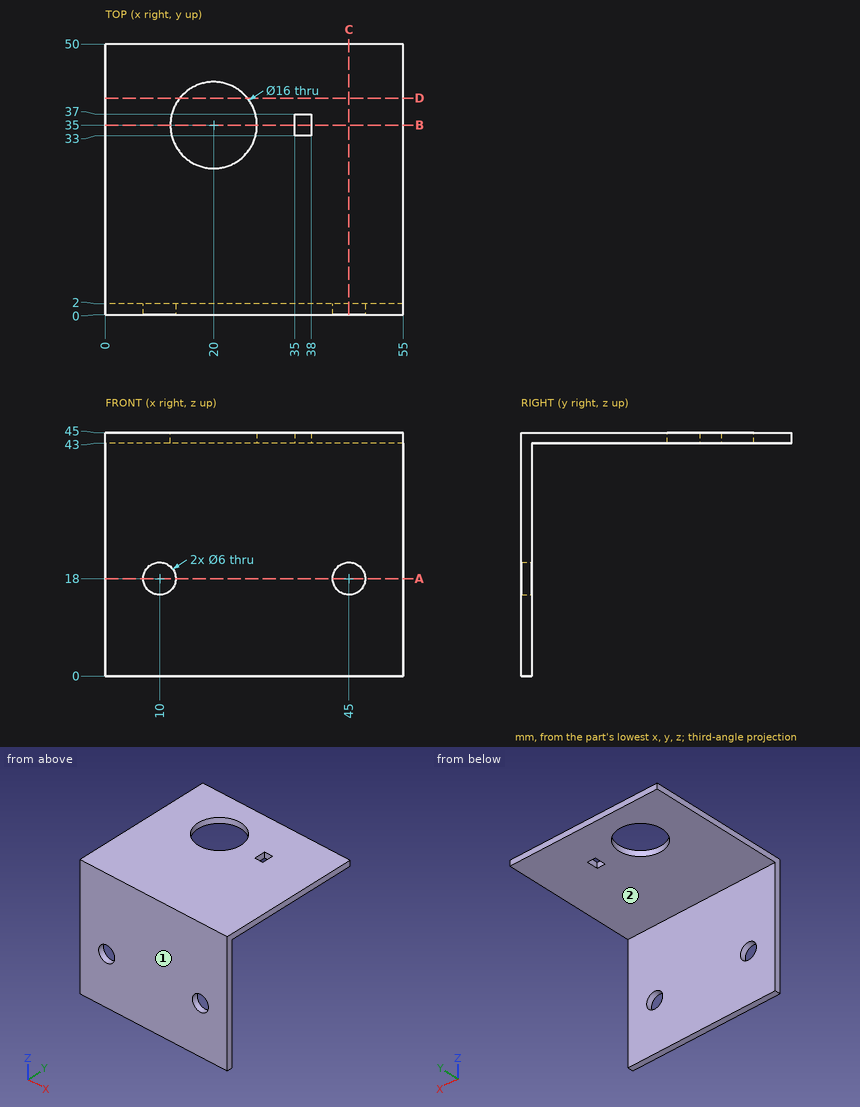
Design review of the part shown in the three views and the two pictorial views. Dimensions are in mm from the part's minimum x, y and z. A direction names the side the tool comes from. Round coordinates to 2 decimals unless told otherwise and drop trailing zeros. Write each loop counter-clockwise with the first axis right and the second up, starting at its lowest first coordinate (ties: lowest second). Pieces come first, ordered by that corner, then holes.
Item 1: Consider section D-D on y = 40. Give the boundary of the cut face in (x, z) (3 decimals), and give its area (3 significant figures).
Item 2: Consider section A-A on z = 18. Give the boundary of the cut face in (x, y).
Item 3: Consider section C-C on x = 45. Give the boundary of the cut face in (y, z).
Item 4: Wall thickness on L1, parallel to X at y = 0.9, z = 18; L2, parallel to Z at x = 10, y = 1; L3, parallel to Y at x = 20, z = 44.6: over which ranges is each line inside the solid? List them lowest first.
Item 5: Consider section B-B on y = 35. Give the boundary of the cut face in (x, z).
Item 6: For the marked faces 1 and 2, list the 3-axis set-ups (+Z, -Z, +X, -X, +Y, -Y) from which the entire face can be reached by the end or side of a thin tool; tool diameter is ignored.
Item 7: For pin 1 Ø10 at (x, z) = (16.5, 28.5) entering from +Y; pin 2 Ø5 at (x, y) = (12, 20.5) entering from -Z, all flat-tipped, find the tip position at first contact; note any pin that passes through.
Check values:
1. outline: (0, 43) - (13.755, 43) - (13.755, 45) - (0, 45) - close; (26.245, 43) - (55, 43) - (55, 45) - (26.245, 45) - close
1. area: 85.0 mm2
2. outline: (0, 0) - (7, 0) - (7, 2) - (0, 2) - close; (13, 0) - (42, 0) - (42, 2) - (13, 2) - close; (48, 0) - (55, 0) - (55, 2) - (48, 2) - close
3. outline: (0, 0) - (2, 0) - (2, 15) - (0, 15) - close; (0, 21) - (2, 21) - (2, 43) - (50, 43) - (50, 45) - (0, 45) - close
4. L1: x = 0 to 7, 13 to 42, 48 to 55
4. L2: z = 0 to 15, 21 to 45
4. L3: y = 0 to 27, 43 to 50
5. outline: (0, 43) - (12, 43) - (12, 45) - (0, 45) - close; (28, 43) - (35, 43) - (35, 45) - (28, 45) - close; (38, 43) - (55, 43) - (55, 45) - (38, 45) - close
6. face 1: +Z, -Z, +X, -X, -Y
6. face 2: -Z, +X, -X, +Y
7. pin 1: stops at y = 2
7. pin 2: stops at z = 43
